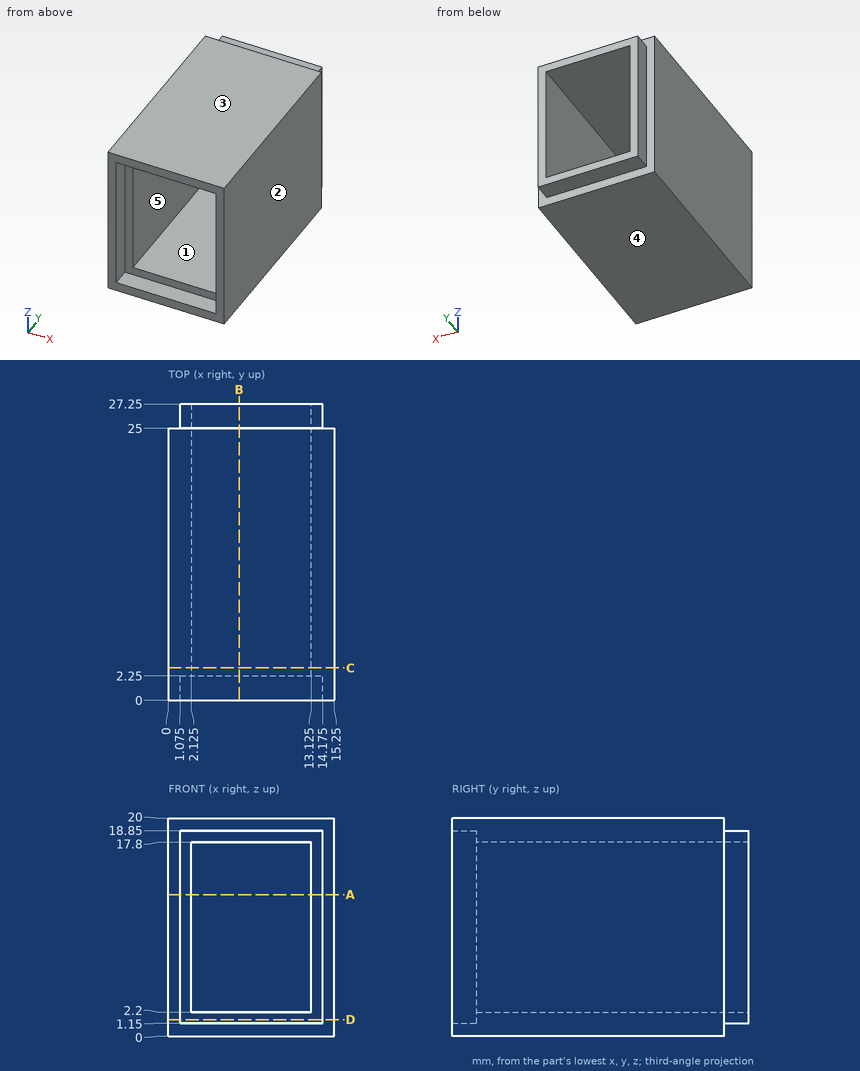
The figure shows three views and two pictorial views of one solid part (mm, origin at its lowest corner). Answer the questions. A direction names the side the tool comes from. Round coordinates to 2 decimals unless told otherwise and drop trailing zeros. Write each loop counter-clockwise with the first axis right and the second up, starting at its lowest first coordinate (ties: lowest second). Pieces come first, ordered by that corner, then holes. Notation, with made-up numbers: (-33.5, 14) - (-27.5, 14) arc R20 cw to (-27.5, 50) - close; hole circle Ø2 at (76.25, 76). An arc over 180 degrees is marked (long way). Use one line per item in the form item = value. Start each with the question number.
Item 1: A tool of negligible diameter and unlimited length cuts with its end or side. For the marked faces 4 and 5, from which of +Z, -Z, +X, -X, +Y, -Y can it reach the whole face along a straight path? Write none if from no direction.
Item 2: Find the intervals of material crossed by line 1 (X direction, y = 15.5, z = 4.25) (3 decimals); line 2 (Z direction, x = 5.75, y = 22); line 3 (X direction, y = 26, z = 15.5) (3 decimals), in increasing order. Write a range as [from, to].
Item 3: A cutting plane is placed at B-B (x = 6.5). Write down the section's boundary in (y, z).
Item 4: A cutting plane is placed at C-C (y = 3). Write down the section's boundary in (x, z) (3 decimals).
Item 5: A cutting plane is placed at D-D (z = 1.5). Write down the section's boundary in (x, y) (3 decimals).
Item 6: Determine the mould class of the marked faces 1, 2 and 3 for opening direction Z: +Z half, -Z half, draft (parallel to the pull), parting line (faces both ways), or undercut.
Item 7: A cutting plane is placed at A-A (z = 13). Write down the section's boundary in (x, y) (3 decimals), plus the area to 3 significant figures.
Item 8: Flat-ended cylindrical pins translate along their axes: pin 1 Ø2 at (x, z) = (5, 6.5) entering from +Y; pin 2 Ø0.7 at (y, z) = (0.5, 11) entering from -X; pin 3 Ø0.7 at (x, y) = (9, 26.5) entering from +Z; pin 4 Ø1.1 at (y, z) = (26, 9.5) entering from -X (3 decimals). Find the tip coordinate at first contact, or state that the pin passes through.
The answers:
q1.face_4 = -Z, +X, -X, +Y, -Y
q1.face_5 = +Y, -Y
q2.line_1 = [0, 2.125], [13.125, 15.25]
q2.line_2 = [0, 2.2], [17.8, 20]
q2.line_3 = [1.075, 2.125], [13.125, 14.175]
q3.outline = (0, 0) - (25, 0) - (25, 1.15) - (27.25, 1.15) - (27.25, 2.2) - (2.25, 2.2) - (2.25, 1.15) - (0, 1.15) - close; (0, 18.85) - (2.25, 18.85) - (2.25, 17.8) - (27.25, 17.8) - (27.25, 18.85) - (25, 18.85) - (25, 20) - (0, 20) - close
q4.outline = (0, 0) - (15.25, 0) - (15.25, 20) - (0, 20) - close; hole (2.125, 2.2) - (13.125, 2.2) - (13.125, 17.8) - (2.125, 17.8) - close
q5.outline = (0, 0) - (1.075, 0) - (1.075, 2.25) - (14.175, 2.25) - (14.175, 0) - (15.25, 0) - (15.25, 25) - (14.175, 25) - (14.175, 27.25) - (1.075, 27.25) - (1.075, 25) - (0, 25) - close
q6.face_1 = undercut
q6.face_2 = draft
q6.face_3 = +Z half
q7.outline = (0, 0) - (1.075, 0) - (1.075, 2.25) - (2.125, 2.25) - (2.125, 27.25) - (1.075, 27.25) - (1.075, 25) - (0, 25) - close; (13.125, 2.25) - (14.175, 2.25) - (14.175, 0) - (15.25, 0) - (15.25, 25) - (14.175, 25) - (14.175, 27.25) - (13.125, 27.25) - close
q7.area = 106 mm^2
q8.pin_1 = through
q8.pin_2 = 0
q8.pin_3 = 18.85
q8.pin_4 = 1.075
